Solid Edge part; units mm, degrees
sketch "Sketch1" plane through (0, 0, 0) normal (1, 0, 0) x (0, 1, 0)
  line L0 (12.6886, 8) -> (10, 8)
  line L1 (10, 8) -> (10, 5)
  line L2 (10, 5) -> (14.1421, 5)
  arc A0 (14.1421, 5) -> (12.6886, -8) centre (0, 0) cw
  line L3 (12.6886, -8) -> (-12.6886, -8)
  arc A1 (-12.6886, -8) -> (-14.1421, 5) centre (0, 0) cw
  line L4 (-10, 5) -> (-14.1421, 5)
  line L5 (-10, 8) -> (-10, 5)
  line L6 (-12.6886, 8) -> (-10, 8)
  arc A2 (-12.6886, 8) -> (12.6886, 8) centre (0, 0) cw
  circle A3 centre (0, 7.7) radius 1.5
  circle A4 centre (7.7, 0) radius 1.5
  circle A5 centre (-7.7, 0) radius 1.5
  dimension "D1" = 10
extrude "Protrusion1" add sketch "Sketch1" against normal blind 3
properties material "Acier"
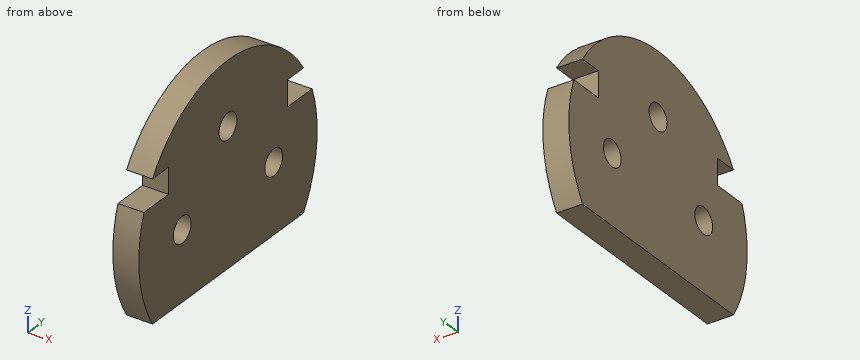
Part model, mm, in its own coordinate system. Round coordinates to 2 decimals unless told otherwise and drop trailing zeros. Write each loop counter-clockwise with the first axis right and the second up, starting at its lowest first coordinate (ties: lowest second). Pieces come first, ordered by that corner, then holes. Notation, with made-up numbers: (71.25, 78) - (90.25, 78) arc R28 cw to (90.25, 114) - close; hole circle Ø10 at (3, 44.25). An arc over 180 degrees is marked (long way). Use CSV: the item, a comma, the result in double quotes.
Item 1: Slice it at A-A, the plane z = 0. Write the cut outline in (x, y).
Results list:
outline,"(-3, -15) - (0, -15) - (0, -9.2) - (-3, -9.2) - close; (-3, -6.2) - (0, -6.2) - (0, 6.2) - (-3, 6.2) - close; (-3, 9.2) - (0, 9.2) - (0, 15) - (-3, 15) - close"
Item 2: Wall check: L1, parallel to Z at x = -2.15, y = 0; L2, parallel to Z at x = -1.7, y = 7.7; L3, parallel to Y at x = -2.65, z = -0.5. Give the ranges that are in metal, low to high.
Results list:
L1,"z = -8 to 6.2, 9.2 to 15"
L2,"z = -8 to -1.5, 1.5 to 12.87"
L3,"y = -14.99 to -9.11, -6.29 to 6.29, 9.11 to 14.99"
Item 3: Flat gauge pins, fed straight in: P1, Ø1.5, axis at x = -0.5, y = 9.5, coming from the +Z side; P2, Ø2.5, axis at y = 0, z = 7.7, coming from the -X side; P3, Ø0.9, axis at x = -1.5, y = -12, coming from the +Z side; P4, Ø1.5, axis at x = -1.5, z = 7, coming from the -Y side. Where does each tip first touch, or does it go through?
Results list:
P1,"stops at z = 12.18"
P2,"passes through"
P3,"stops at z = 9.57"
P4,"stops at y = -10"
Item 4: Slice it at D-D, the plane y = 5. Write the cut outline in (x, z), then the cut area to 3 significant figures.
Results list:
outline,"(-3, -8) - (0, -8) - (0, 14.14) - (-3, 14.14) - close"
area,"66.4 mm²"
Item 5: Slice it at B-B, the plane x = -1.7. Write the cut outline in (y, z).
Results list:
outline,"(-14.14, 5) arc R15 ccw to (-12.69, -8) - (12.69, -8) arc R15 ccw to (14.14, 5) - (10, 5) - (10, 8) - (12.69, 8) arc R15 ccw to (-12.69, 8) - (-10, 8) - (-10, 5) - close; hole circle Ø3 at (-7.7, 0); hole circle Ø3 at (0, 7.7); hole circle Ø3 at (7.7, 0)"
Item 6: Slice it at C-C, the plane y = 0. Write the cut outline in (x, z).
Results list:
outline,"(-3, -8) - (0, -8) - (0, 6.2) - (-3, 6.2) - close; (-3, 9.2) - (0, 9.2) - (0, 15) - (-3, 15) - close"
